```python
from build123d import *

# Parameters (mm, degrees)
SKETCH001_R      = 2.5
EXTRUDE001_DEPTH = 2
ARRAY_X_COUNT    = 3
ARRAY_X_PITCH    = 10
ARRAY_Y_COUNT    = 2
ARRAY_Y_PITCH    = 10
SKETCH_R         = 5
EXTRUDE_DEPTH    = 2


with BuildPart() as array:
    # Sketch001 (on Sketch) → Extrude001 (new body)
    with BuildSketch(Plane.XY):
        with Locations((6, 9)):
            Circle(SKETCH001_R)
    extrude(amount=EXTRUDE001_DEPTH)

    # Array X: Array ×3


with BuildPart() as array_1:
    add(array.part)
    with Locations(*[(i * ARRAY_X_PITCH, 0, 0) for i in range(1, ARRAY_X_COUNT)]):
        add(array.part)

    # Array Y: Array ×2


with BuildPart() as array_2:
    add(array_1.part)
    with Locations(*[(0, -i * ARRAY_Y_PITCH, 0) for i in range(1, ARRAY_Y_COUNT)]):
        add(array_1.part)


with BuildPart() as cut:
    # Sketch → Extrude (new body)
    with BuildSketch(Plane.XY):
        with BuildLine():
            ThreePointArc((0, 8.660254), (-15, 0), (0, -8.660254))
            Line((0, -17.601841), (0, -8.660254))
            Line((29.294832, -17.601841), (0, -17.601841))
            Line((29.294832, 17.601841), (29.294832, -17.601841))
            Line((0, 17.601841), (29.294832, 17.601841))
            Line((0, 8.660254), (0, 17.601841))
        make_face()
        with Locations((-5, 0)):
            Circle(SKETCH_R, mode=Mode.SUBTRACT)
    extrude(amount=EXTRUDE_DEPTH)

    # Cut: cut Array
    add(array_2.part, mode=Mode.SUBTRACT)


solid = cut.part
```
Model file for the job. Use its own axes, mm. Coordinates: 2 decimals unless noted, no trailing zeros. Loops run counter-clockwise (first coordinate to the right, second up) from the corner with the lowest first, then second, coordinate; pieces in that order, holes last. Notation, with made-up numbers: M -20.75,32 L 15.25,32 A17 ccw 15.25,36 Z; hole C 4,-8 d1. An arc over 180 degrees is marked long. Use CSV: the item, a comma, the result in double quotes. Start each with the question number.
1. Band-saw the part on B-B, the plane z = 0.9. List the corners of the cut face in (x, y).
2. Band-saw the part on A-A, the plane x = -5. List the corners of the cut face in (y, z).
3. Two-plate mould, pull along X, no slides. Class faces 1 (the cylindrical face through (24, -2.5, 1)), 2 (the flat face through (29.295, 0, 1)), 3 (the flat face through (14, 17.602, 1)): pulls with the +X half, pulls with the -X half, needs draft (parallel to the pull), parting line crosses it, or undercut.
4. Band-saw the part on D-D, the plane y = -4. List the corners of the cut face in (x, z), then the cut area to 3 significant figures.
5. Flat gauge pins, fed straight in: pin 1 (3 mm diameter, centred on x = 26, y = 9, fed in from +Z); pin 2 (1 mm diameter, centred on y = 14, z = 1, fed in from -X). Where does each tip first touch, or does it go through?
6. Band-saw the part on C-C, the plane x = 26. List the corners of the cut face in (y, z).
7. Probe probe 1 along Y at (x, z) = (16, 0.6); probe 2 along Y at (x, z) = (25, 1.9); probe 3 along X at (y, z) = (1, 0.2). List the from-to ranges inside material, lowest first. Write a range as [from, to].
Entries:
1,outline,"M 0,-17.6 L 29.29,-17.6 L 29.29,17.6 L 0,17.6 L 0,8.66 A10 ccw long 0,-8.66 Z; hole C -5,0 d10; hole C 6,-1 d5; hole C 6,9 d5; hole C 16,-1 d5; hole C 16,9 d5; hole C 26,-1 d5; hole C 26,9 d5"
2,outline,"M -10,0 L -5,0 L -5,2 L -10,2 Z; M 5,0 L 10,0 L 10,2 L 5,2 Z"
3,face 1,"undercut"
3,face 2,"pulls with the +X half"
3,face 3,"needs draft"
4,outline,"M -14.17,0 L -8,0 L -8,2 L -14.17,2 Z; M -2,0 L 29.29,0 L 29.29,2 L -2,2 Z"
4,area,"74.9 mm2"
5,pin 1,"passes through"
5,pin 2,"stops at x = 0"
6,outline,"M -17.6,0 L -3.5,0 L -3.5,2 L -17.6,2 Z; M 1.5,0 L 6.5,0 L 6.5,2 L 1.5,2 Z; M 11.5,0 L 17.6,0 L 17.6,2 L 11.5,2 Z"
7,probe 1,"y = [-17.6, -3.5], [1.5, 6.5], [11.5, 17.6]"
7,probe 2,"y = [-17.6, -3.29], [1.29, 6.71], [11.29, 17.6]"
7,probe 3,"x = [-14.95, -9.9], [-0.1, 4.5], [7.5, 14.5], [17.5, 24.5], [27.5, 29.29]"
